```python
from build123d import *

# Parameters (mm, degrees)
SKETCH1_W           = 317.5
SKETCH1_H           = 101.6
BOSS_EXTRUDE1_DEPTH = 8.0518
BOSS_EXTRUDE2_START = 8.0518
SKETCH2_W           = 317.5
SKETCH2_H           = 8.128
BOSS_EXTRUDE2_DEPTH = 103.378
BOSS_EXTRUDE3_START = 8.0518
SKETCH3_W           = 9.525
SKETCH3_H           = 46.5328
BOSS_EXTRUDE3_DEPTH = 76.9874
BOSS_EXTRUDE4_START = 8.0518
SKETCH3_3_W         = 9.525
SKETCH3_3_H         = 46.5328
BOSS_EXTRUDE4_DEPTH = 76.1746
BOSS_EXTRUDE5_DEPTH = 317.5


with BuildPart() as part:
    # Sketch1 → Boss-Extrude1 (new body)
    with BuildSketch(Plane(origin=(0, 0, 0), x_dir=(1, 0, 0), z_dir=(0, 1, 0))):
        with Locations((158.75, 50.8)):
            Rectangle(SKETCH1_W, SKETCH1_H)
    extrude(amount=BOSS_EXTRUDE1_DEPTH)

    # Sketch2 → Boss-Extrude2 (add)
    with BuildSketch(Plane(origin=(0, 0, 0), x_dir=(1, 0, 0), z_dir=(0, 1, 0)).offset(BOSS_EXTRUDE2_START)):
        with Locations((158.75, 50.5968)):
            Rectangle(SKETCH2_W, SKETCH2_H)
    extrude(amount=BOSS_EXTRUDE2_DEPTH)

    # Sketch3 → Boss-Extrude3 (add)
    with BuildSketch(Plane(origin=(0, 0, 0), x_dir=(1, 0, 0), z_dir=(0, 1, 0)).offset(BOSS_EXTRUDE3_START)):
        with Locations((6.6675, 23.2664)):
            Rectangle(SKETCH3_W, SKETCH3_H)
    extrude(amount=BOSS_EXTRUDE3_DEPTH)

    # Sketch3<3> → Boss-Extrude4 (add)
    with BuildSketch(Plane(origin=(0, 0, 0), x_dir=(1, 0, 0), z_dir=(0, 1, 0)).offset(BOSS_EXTRUDE4_START)):
        with Locations((165.1635, 23.2664)):
            Rectangle(SKETCH3_3_W, SKETCH3_3_H)
    extrude(amount=BOSS_EXTRUDE4_DEPTH)

    # Sketch4 → Boss-Extrude5 (add)
    with BuildSketch(Plane(origin=(0, 0, 0), x_dir=(0, 0, -1), z_dir=(1, 0, 0))):
        with BuildLine():
            Line((61.6458, 8.0518), (54.6608, 8.0518))
            Line((54.6608, 8.0518), (54.6608, 15.0368))
            ThreePointArc((54.6608, 15.0368), (59.20078128, 12.59178128), (61.6458, 8.0518))
        make_face()
    extrude(amount=BOSS_EXTRUDE5_DEPTH)


solid = part.part
```
Build history of the part. All positions in model axes, mm. A direction names the side the tool comes from. Round coordinates to 2 decimals unless told otherwise and drop trailing zeros. Order: outer loops, then holes, each group sorted by start corner. A loop starts at its lowest first (then second) coordinate and runs counter-clockwise, first axis right, second up. Notation, with made-up numbers: (-32.75, 74.25) - (5.25, 74.25) arc R32 ccw to (5.25, 106.25) - close; hole circle Ø5 at (85, 22). An arc over 180 degrees is marked (long way). Use a Markdown table: item, result.
1) Tool access for faces 1 (the face through (169.926, 46, -23)), 2 (the face through (160.401, 46, -23)), 3 (the face through (7, 85.039, -24)): list every direction of +Z, -Z, +X, -X, +Y, -Y with a clear straight run to the whole face (end or side of a thin tool).
Recorded:
| item | result |
|---|---|
| face 1 | +Z, +X, +Y |
| face 2 | +Z, +Y |
| face 3 | +Z, +X, -X, +Y |
2) Saw through at C-C on y = 74. Write the cut outline in (x, z) (3 decimals), and give its area (3 significant figures).
Recorded:
| item | result |
|---|---|
| outline | (0, -54.661) - (317.5, -54.661) - (317.5, -46.533) - (169.926, -46.533) - (169.926, 0) - (160.401, 0) - (160.401, -46.533) - (11.43, -46.533) - (11.43, 0) - (1.905, 0) - (1.905, -46.533) - (0, -46.533) - close |
| area | 3,470 mm² |
3) Saw through at D-D on x = 121. Write the cut outline in (y, z), and give its area (3 significant figures).
Recorded:
| item | result |
|---|---|
| outline | (0, -101.6) - (8.05, -101.6) - (8.05, -61.65) arc R8.97 ccw to (15.04, -54.66) - (111.43, -54.66) - (111.43, -46.53) - (8.05, -46.53) - (8.05, 0) - (0, 0) - close |
| area | 1,690 mm² |
4) Wall check: L1, parallel to X at y = 60.5, z = -21 (3 decimals); L2, parallel to Y at x = 206, z = -91.5; L3, parallel to Z at x = 193.5, y = 98.5. Give the ranges that are in metal, low to high.
Recorded:
| item | result |
|---|---|
| L1 | x = 1.905 to 11.43, 160.401 to 169.926 |
| L2 | y = 0 to 8.05 |
| L3 | z = -54.66 to -46.53 |
5) Saw through at A-A on z = -28. Write the cut outline in (x, y) (3 decimals), and give its area (3 significant figures).
Recorded:
| item | result |
|---|---|
| outline | (0, 0) - (317.5, 0) - (317.5, 8.052) - (169.926, 8.052) - (169.926, 84.226) - (160.401, 84.226) - (160.401, 8.052) - (11.43, 8.052) - (11.43, 85.039) - (1.905, 85.039) - (1.905, 8.052) - (0, 8.052) - close |
| area | 4,020 mm² |
6) Flat gauge pins, fed straight in: pin 1 Ø3 at (x, z) = (163, -12) entering from +Y; pin 2 Ø2 at (y, z) = (38.5, -35.5) entering from -X (3 decimals); pin 3 Ø23.5 at (x, z) = (97, -25) entering from +Y; pin 4 Ø5 at (x, z) = (219, -32) entering from -Y. Where does each tip first touch, or does it go through?
Recorded:
| item | result |
|---|---|
| pin 1 | stops at y = 84.23 |
| pin 2 | stops at x = 1.905 |
| pin 3 | stops at y = 8.05 |
| pin 4 | stops at y = 0 |
7) Saw through at B-B on x = 166.5. Write the cut outline in (y, z).
Recorded:
| item | result |
|---|---|
| outline | (0, -101.6) - (8.05, -101.6) - (8.05, -61.65) arc R8.97 ccw to (15.04, -54.66) - (111.43, -54.66) - (111.43, -46.53) - (84.23, -46.53) - (84.23, 0) - (0, 0) - close |
8) Pull direction X, two halves, no side cores. Call faces 4 (the face through (11.43, 46, -23)), 5 (the face through (317.5, 31, -51)), 6 (the face through (1.905, 46, -23)): pulls with the +X half, pulls with the -X half, needs draft (parallel to the pull), parting line crosses it, or undercut.
Recorded:
| item | result |
|---|---|
| face 4 | undercut |
| face 5 | pulls with the +X half |
| face 6 | pulls with the -X half |
